from build123d import *

# Parameters (mm, degrees)
F0_W        = 29.972
F0_H        = 50.038
F1_DEPTH    = 64.262
F2_SIZE     = 25.4
F3_DEPTH    = 28.194
F4_T1_DEPTH = 102.362
F5_R        = 1.7813508629
F6_DEPTH    = 12.192
F7_W        = 49.9822117854
F7_H        = 16.4834968746
F8_DEPTH    = 137.16
F9_R        = 3.81


# Not quite as in the source:
# - a fillet or chamfer that OpenCascade refuses, or shapes differently, is made with other operations: its cross-section is extruded or revolved along the edge and cut away or added


with BuildPart() as f1:
    # F0 (on Right) → F1 (new body)
    with BuildSketch(Plane.YZ):
        with Locations((-12.6866316661, -8.6694222925)):
            Rectangle(F0_W, F0_H)
    extrude(amount=F1_DEPTH)

    # F2
    f2_edges = [f1.edges().sort_by_distance(p)[0] for p in [
        (32.131, -27.672632, 16.349578),
    ]]
    chamfer(f2_edges, length=F2_SIZE)

    # F3 (add): a face of the model
    f3_faces = [f1.faces().sort_by_distance(p)[0] for p in [
        (32.131, -27.6726316661, -21.3694222925),
    ]]
    extrude(f3_faces, amount=F3_DEPTH)

    # F4: fillet of radius 7.62 on 4 edges, made by hand

    # F4_s2 → F4_t1 (cut)
    with BuildSketch(Plane.YZ.offset(-19.05)):
        with BuildLine():
            ThreePointArc((-48.2466316661, -33.6884222925), (-53.6347853387, -31.4565759651), (-55.8666316661, -26.0684222925))
            Line((-55.8666316661, -26.0684222925), (-55.8666316661, -33.6884222925))
            Line((-55.8666316661, -33.6884222925), (-48.2466316661, -33.6884222925))
        make_face()
        with BuildLine():
            ThreePointArc((-55.8666316661, -16.6704222925), (-53.6347853387, -11.2822686198), (-48.2466316661, -9.0504222925))
            Line((-48.2466316661, -9.0504222925), (-55.8666316661, -9.0504222925))
            Line((-55.8666316661, -9.0504222925), (-55.8666316661, -16.6704222925))
        make_face()
    extrude(amount=F4_T1_DEPTH, mode=Mode.SUBTRACT)

    # F5 (on face) → F6 (cut)
    with BuildSketch(Plane(origin=(0, -9.3111046868, 9.3111046868), x_dir=(1, 0, 0), z_dir=(0, -0.7071067812, 0.7071067812))):
        with Locations((35.1360822096, -11.1896051094)):
            Circle(F5_R)
        with Locations((49.9720936641, 0.6819777191)):
            Circle(F5_R)
        with Locations((33.6671667174, 0.486287754)):
            Circle(F5_R)
        with Locations((18.350715749, -11.7116672918)):
            Circle(F5_R)
    extrude(amount=-F6_DEPTH, mode=Mode.SUBTRACT)

    # F7 (on face) → F8 (cut)
    with BuildSketch(Plane.YZ.offset(64.262)):
        with Locations((-26.5206474578, -21.5896144509)):
            Rectangle(F7_W, F7_H)
    extrude(amount=-F8_DEPTH, mode=Mode.SUBTRACT)

    # F9
    f9_edges = [f1.edges().sort_by_distance(p)[0] for p in [
        (32.131, -51.511753, -13.347866),
        (32.131, -51.511753, -29.831363),
    ]]
    fillet(f9_edges, radius=F9_R)


solid = f1.part
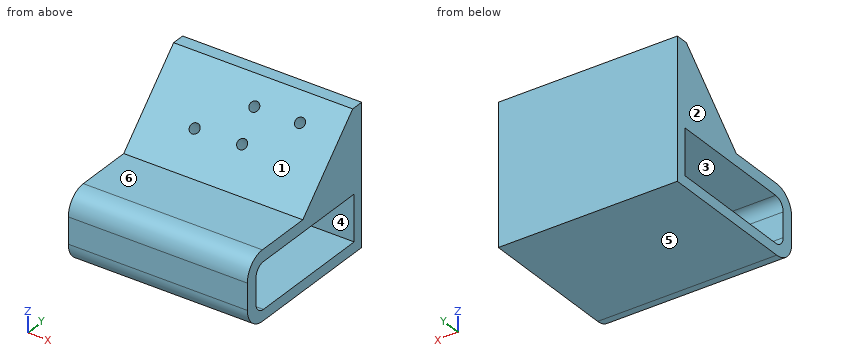
Model file for the job. Use its own axes, mm. Face numbers are marked on the shaded views. A direction names the side the tool comes from. Round coordinates to 2 decimals unless told otherwise and drop trailing zeros. Order: outer loops, then holes, each group sorted by start corner. A loop starts at its lowest first (then second) coordinate and runs counter-clockwise, first axis right, second up.
(1) Pin check, flat tips, straight feed: pin 1 (6 mm diameter, centred on x = 47.5, z = 9.5, fed in from -Y); pin 2 (8 mm diameter, centred on x = 11, z = 0.5, fed in from -Y); pin 3 (22.5 mm diameter, centred on x = 40.5, y = -42, fed in from +Z). Stop position of each tip, or through.
(2) Band-saw the part on A-A (x = 10.5). List the corners of the cut face in (y, z).
(3) Band-saw the part on C-C (z = -15). List the corners of the cut face in (x, y), then the cut area to 3 significant figures.
(4) Drill centre lines: line 1 (X direction, y = -2.5, z = 3.5); line 2 (Z direction, x = 28, y = -46.5); line 3 (Y direction, x = 26, z = -26). Where is each one in solid material? Low to high.
(5) Band-saw the part on B-B (y = -30). List the corners of the cut face in (x, z).
(6) 3-axis set-ups, long thin cutter, end or side, ignore diameter. For the marked faces 4, 5 and 6: which of +Z, -Z, +X, -X, +Y, -Y reach the whole face in a straight line?
(7) Pull direction Y, two halves, no side cores. Call the marked faces 1, 2 and 3: released by +Y, released by -Y, zero draft, split by the parting line, or undercut.
(8) Band-saw the part on D-D (y = -5). Give the number of separate pieces and of enclosed holes in the cut face, then the cut area to 3 significant figures.
Verdict:
1. pin 1: stops at y = -12.12
1. pin 2: stops at y = -22.12
1. pin 3: stops at z = -9.05
2. outline: (-55.87, -26.07) arc R7.62 ccw to (-48.25, -33.69) - (2.3, -33.69) - (2.3, 16.35) - (-2.27, 16.35) - (-27.67, -9.05) - (-48.25, -9.05) arc R7.62 ccw to (-55.87, -16.67) - close; hole (-51.51, -26.02) arc R3.81 ccw to (-47.7, -29.83) - (-1.53, -29.83) - (-1.53, -13.35) - (-47.7, -13.35) arc R3.81 ccw to (-51.51, -17.16) - close
3. outline: (0, -55.68) - (64.26, -55.68) - (64.26, -50.84) - (0, -50.84) - close; (0, -1.53) - (64.26, -1.53) - (64.26, 2.3) - (0, 2.3) - close
3. area: 557 mm2
4. line 1: x = 0 to 31.9, 35.43 to 48.19, 51.75 to 64.26
4. line 2: z = -33.69 to -29.83, -13.35 to -9.05
4. line 3: y = -55.87 to -51.51, -1.53 to 2.3
5. outline: (0, -33.69) - (64.26, -33.69) - (64.26, -29.83) - (0, -29.83) - close; (0, -13.35) - (64.26, -13.35) - (64.26, -9.05) - (0, -9.05) - close
6. face 4: +X, -X
6. face 5: -Z, +X, -X, +Y, -Y
6. face 6: +Z, +X, -X, -Y
7. face 1: released by -Y
7. face 2: zero draft
7. face 3: undercut
8. separate pieces: 2
8. enclosed holes: 2
8. area: 1,950 mm2
